Geometry check sheet. Reference: the model listing, model coordinates, mm. A direction names the side the tool comes from. Give positions to 0.01 mm unless a question says otherwise; leave off trailing zeros. Loops run counter-clockwise (first coordinate to the right, second up) from the corner with the lowest first, then second, coordinate; pieces in that order, holes last.
1. Cross-section at B-B, the plane y = 0. Record the cut outline in (x, z).
2. Tool access check on faces 4 (the cylindrical face through (-0.221, -34.493, -1.479)), 5 (the flat face through (25, -31.5, -1)), 6 (the flat face through (25, 31.5, -1)). Record the directions out of +Z, -Z, +X, -X, +Y, -Y that give a thin tool (end or side, any length) a straight path to the whole face; none if there is none.
3. Material ranges on L1, parallel to Y at x = 0, z = -1.9; L2, parallel to Y at x = 21.7, z = -1.4; L3, parallel to X at y = 1, z = -1.4, recorded low to high.
4. Cross-section at A-A, the plane x = 21.7. Record the cut outline in (y, z), plus the area to 3 significant figures.
5. Cross-section at C-C, the plane x = 0. Record the cut outline in (y, z).
6. Cross-section at D-D, the plane z = -1.2. State how many separate pieces and enclosed holes the cut face has, plus the area to 3 significant figures.
7. Release check for a two-part mould opening along Y. For faces 1 (the cylindrical face through (4.353, -31.975, -1.521)), 2 (the flat face through (27, 0, 0)), 3 (the cylindrical face through (2.285, 3.584, -1.479)) record: +Y half, -Y half, draft (parallel to the pull), parting line (faces both ways), or undercut.
8. Go/stop test with flat-tipped pins: pin 1 Ø0.9 at (x, z) = (20, -2) entering from +Y; pin 2 Ø1.5 at (x, z) = (64.5, -1.5) entering from +Y; pin 3 Ø1 at (x, z) = (43.5, -2) entering from -Y. Record where each tip stops, or that it passes through.
from build123d import *

# Parameters (mm, degrees)
SKETCH1_R           = 4
SKETCH1_R_2         = 4.25
SKETCH1_R_3         = 1.5
BOSS_EXTRUDE1_DEPTH = 3
FILLET1_R           = 5


with BuildPart() as part:
    # Sketch1 → Boss-Extrude1 (new body)
    with BuildSketch(Plane.XY):
        with BuildLine():
            Line((47.025062814, 31.5), (3.464101615, 31.5))
            ThreePointArc((3.464101615, 31.5), (-0.097423396, 34.498643835), (-3.486558103, 31.306451613))
            ThreePointArc((-3.486558103, 31.306451613), (-21.727681967, 22.80696903), (-31.100806452, 4.998983703))
            ThreePointArc((-31.100806452, 4.998983703), (-26, 0), (-31.100806452, -4.998983703))
            ThreePointArc((-31.100806452, -4.998983703), (-21.727681967, -22.80696903), (-3.486558103, -31.306451613))
            ThreePointArc((-3.486558103, -31.306451613), (-0.097423396, -34.498643835), (3.464101615, -31.5))
            Line((3.464101615, -31.5), (47.025062814, -31.5))
            ThreePointArc((47.025062814, -31.5), (51.800041427, -26.003999943), (56.998983703, -31.100806452))
            ThreePointArc((56.998983703, -31.100806452), (74.80696903, -21.727681967), (83.306451613, -3.486558103))
            ThreePointArc((83.306451613, -3.486558103), (86.5, 0), (83.306451613, 3.486558103))
            ThreePointArc((83.306451613, 3.486558103), (74.80696903, 21.727681967), (56.998983703, 31.100806452))
            ThreePointArc((56.998983703, 31.100806452), (51.800041427, 26.003999943), (47.025062814, 31.5))
        make_face()
        with Locations((35.75, -19.75)):
            Circle(SKETCH1_R, mode=Mode.SUBTRACT)
        Circle(SKETCH1_R_2, mode=Mode.SUBTRACT)
        with Locations((21.7, 0)):
            Circle(SKETCH1_R_3, mode=Mode.SUBTRACT)
    extrude(amount=-BOSS_EXTRUDE1_DEPTH)

    # Fillet1
    fillet1_edges = [part.edges().sort_by_distance(p)[0] for p in [
        (3.464101615, 31.5, -1.5),
        (47.025062814, 31.5, -1.5),
        (56.998983703, 31.100806452, -1.5),
        (83.306451613, 3.486558103, -1.5),
        (83.306451613, -3.486558103, -1.5),
        (56.998983703, -31.100806452, -1.5),
        (47.025062814, -31.5, -1.5),
        (3.464101615, -31.5, -1.5),
        (-3.486558103, -31.306451613, -1.5),
        (-31.100806452, -4.998983703, -1.5),
        (-31.100806452, 4.998983703, -1.5),
        (-3.486558103, 31.306451613, -1.5),
    ]]
    fillet(fillet1_edges, radius=FILLET1_R)


solid = part.part
Result:
1. outline: (-26, -3) - (-4.25, -3) - (-4.25, 0) - (-26, 0) - close; (4.25, -3) - (20.2, -3) - (20.2, 0) - (4.25, 0) - close; (23.2, -3) - (86.5, -3) - (86.5, 0) - (23.2, 0) - close
2. face 4: +Z, -Z, -Y
2. face 5: +Z, -Z, +X, -Y
2. face 6: +Z, -Z, +X, +Y
3. L1: y = -34.5 to -4.25, 4.25 to 34.5
3. L2: y = -31.5 to -1.5, 1.5 to 31.5
3. L3: x = -26.1 to -4.13, 4.13 to 20.58, 22.82 to 86.35
4. outline: (-31.5, -3) - (-1.5, -3) - (-1.5, 0) - (-31.5, 0) - close; (1.5, -3) - (31.5, -3) - (31.5, 0) - (1.5, 0) - close
4. area: 180 mm2
5. outline: (-34.5, -3) - (-4.25, -3) - (-4.25, 0) - (-34.5, 0) - close; (4.25, -3) - (34.5, -3) - (34.5, 0) - (4.25, 0) - close
6. separate pieces: 1
6. enclosed holes: 3
6. area: 6,180 mm2
7. face 1: -Y half
7. face 2: draft
7. face 3: undercut
8. pin 1: stops at y = 31.5
8. pin 2: stops at y = 29.23
8. pin 3: stops at y = -31.5
